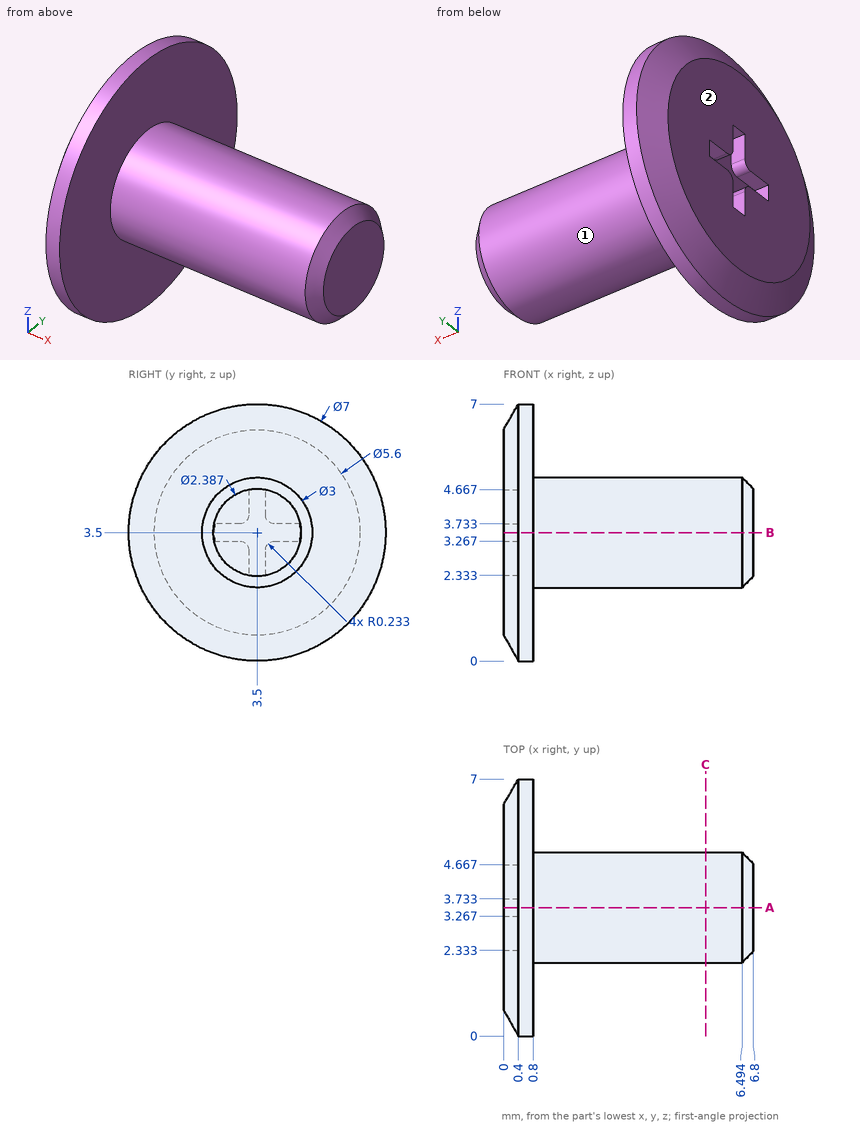
Geometry check sheet. Reference: drawing and pictorial views, mm from the part's lowest x, y, z. A direction names the side the tool comes from. Give positions to 0.01 mm unless a question says otherwise; leave off trailing zeros. Order: outer loops, then holes, each group sorted by start corner. A loop starts at its lowest first (then second) coordinate and runs counter-clockwise, first axis right, second up. Notation, with made-up numbers: M -20.5,37.25 L -13.5,37.25 A18 cw -13.5,72.25 Z; hole C -38.5,79 d11. An arc over 180 degrees is marked long. Answer as a JSON object with one key per item and string values. Group by question number.
1) Scan lines: line 1 along X through (y, z) = (1.25, 4); line 2 along Y through (x, z) = (5.25, 3.5); line 3 along X through (y, z) = (0.5, 2) (1 decimal). Record each from-to range of solid material in increasing order. Write a range as [from, to].
2) Cross-section at C-C (x = 5.5). Enter the section's corners in (y, z).
3) Depth check by flat-ended pin: pin 1 Ø1 at (x, y) = (6, 3.5) entering from -Z; pin 2 Ø1.2 at (y, z) = (4, 3.5) entering from -X; pin 3 Ø1 at (x, z) = (4.5, 3) entering from +Y; pin 4 Ø1 at (x, y) = (4, 1) entering from +Z. Enter the tip coordinate at first touch or a pass-through.
4) Cross-section at A-A (y = 3.5). Enter the section's corners in (x, z), then the cut area to 3 significant figures.
5) Access from +Z, -Z, +X, -X, +Y, -Y to the whole of each face (thin tool, end or side, straight path). Record for the marked faces 1 and 2.
Result sheet:
{
 "1": {"line 1": "x = [0, 0.8]", "line 2": "y = [2, 5]", "line 3": "x = [0.3, 0.8]"},
 "2": {"outline": "C 3.5,3.5 d3"},
 "3": {"pin 1": "stops at z = 2", "pin 2": "stops at x = 0", "pin 3": "stops at y = 5", "pin 4": "passes through"},
 "4": {"outline": "M 0,0.7 L 0.4,0 L 0.8,0 L 0.8,2 L 6.49,2 L 6.8,2.31 L 6.8,4.69 L 6.49,5 L 0.8,5 L 0.8,7 L 0.4,7 L 0,6.3 L 0,4.67 L 0.4,4.67 L 0.4,2.33 L 0,2.33 Z", "area": "22.3 mm2"},
 "5": {"face 1": "+X", "face 2": "+Z, -Z, -X, +Y, -Y"}
}
